from build123d import *

# Parameters (mm, degrees)
SKIZZE1_W                       = 120
SKIZZE1_H                       = 123
AUFSATZ_LINEAR_AUSTRAGEN1_DEPTH = 46
SKIZZE2_R                       = 3.007311743
AUFSATZ_LINEAR_AUSTRAGEN2_DEPTH = 10


with BuildPart() as part:
    # Skizze1 → Aufsatz-Linear austragen1 (new body)
    with BuildSketch(Plane(origin=(0, 0, 0), x_dir=(1, 0, 0), z_dir=(0, 1, 0))):
        Rectangle(SKIZZE1_W, SKIZZE1_H)
    extrude(amount=AUFSATZ_LINEAR_AUSTRAGEN1_DEPTH)

    # Skizze2 → Aufsatz-Linear austragen2 (add)
    with BuildSketch(Plane.XY.offset(61.5)):
        with Locations(Location((-26.717027071, 22.669789553, 0), (0, 0, 180))):
            Circle(SKIZZE2_R)
        with Locations(Location((27.737677543, 22.669789553, 0), (0, 0, 180))):
            Circle(SKIZZE2_R)
    extrude(amount=AUFSATZ_LINEAR_AUSTRAGEN2_DEPTH)


solid = part.part
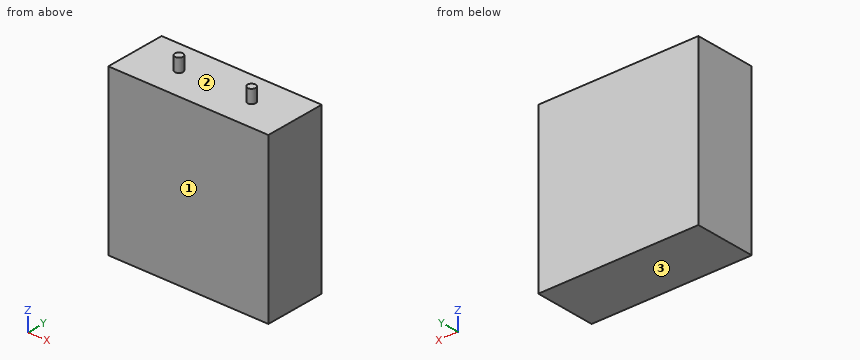
Design review of the part built by this model. Coordinates are the model's own, in mm. Face numbers are marked on the shaded views. Coordinates: 2 decimals unless noted, no trailing zeros. Loops run counter-clockwise (first coordinate to the right, second up) from the corner with the lowest first, then second, coordinate; pieces in that order, holes last.
Item 1: Clearance check with a flat-ended pin moving along its axis: pin 1 (2 mm diameter, centred on x = 11.5, y = 41, fed in from +Z). State where the tip first meets the part, or that it passes through.
Completed:
pin 1: stops at z = 61.5
Item 2: Draft analysis for pull direction Z (two halves, no side actions). For the marked faces 1, 2 and 3, state which applies: pulls with the +Z half, pulls with the -Z half, needs draft (parallel to the pull), parting line crosses it, or undercut.
Completed:
face 1: needs draft
face 2: pulls with the +Z half
face 3: pulls with the -Z half
Item 3: Add section A-A (y = 4). Write out the cut boundary in (x, z).
Completed:
outline: (-60, -61.5) - (60, -61.5) - (60, 61.5) - (-60, 61.5) - close
Item 4: Add section B-B (x = -48.5). Write out the cut boundary in (y, z), and give its area (3 significant figures).
Completed:
outline: (0, -61.5) - (46, -61.5) - (46, 61.5) - (0, 61.5) - close
area: 5,660 mm2
Item 5: Wall thickness on L1, parallel to Z at x = -33.5, y = 19.5: over which ranges is the line inside the solid? List them lowest first.
Completed:
L1: z = -61.5 to 61.5
